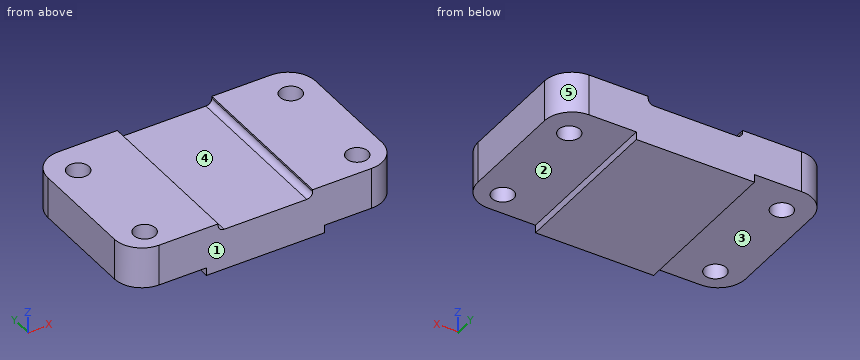
from build123d import *

# Parameters (mm, degrees)
F0_W     = 44
F0_H     = 82
F0_R     = 5.5
F0_W_2   = 48
F1_DEPTH = 12.5
F2_R     = 14
F3_W     = 48
F3_H     = 4
F4_DEPTH = 82.001
F5_R     = 3
F6_W     = 38
F6_H     = 4
F7_DEPTH = 82.001


with BuildPart() as f1:
    # F0 (on Top) → F1 (new body, symmetric)
    with BuildSketch(Plane.XY):
        with Locations((22, 41)):
            Rectangle(F0_W, F0_H)
        with Locations((14, 11.8173863739)):
            Circle(F0_R, mode=Mode.SUBTRACT)
        with Locations((14, 65.8173863739)):
            Circle(F0_R, mode=Mode.SUBTRACT)
        with Locations((68, 41)):
            Rectangle(F0_W_2, F0_H)
        with Locations((114, 41)):
            Rectangle(F0_W, F0_H)
        with Locations((122, 11.8173863739)):
            Circle(F0_R, mode=Mode.SUBTRACT)
        with Locations((122, 65.8173863739)):
            Circle(F0_R, mode=Mode.SUBTRACT)
    extrude(amount=F1_DEPTH, both=True)

    # F2
    f2_edges = [f1.edges().sort_by_distance(p)[0] for p in [
        (0, 82, 0),
        (136, 82, 0),
        (136, 0, 0),
        (0, 0, 0),
    ]]
    fillet(f2_edges, radius=F2_R)

    # F3 (on face) → F4 (cut, through all)
    with BuildSketch(Plane.XZ):
        with Locations((68, 10.5)):
            Rectangle(F3_W, F3_H)
    extrude(amount=-F4_DEPTH, mode=Mode.SUBTRACT)

    # F5
    f5_edges = [f1.edges().sort_by_distance(p)[0] for p in [
        (44, 41, 8.5),
        (92, 41, 8.5),
    ]]
    fillet(f5_edges, radius=F5_R)

    # F6 (on face) → F7 (cut, through all)
    with BuildSketch(Plane.XZ):
        with Locations((117, -10.5)):
            Rectangle(F6_W, F6_H)
        with Locations((19, -10.5)):
            Rectangle(F6_W, F6_H)
    extrude(amount=-F7_DEPTH, mode=Mode.SUBTRACT)


solid = f1.part
Geometry: final body of the model. Coordinates: model frame, mm. Face numbers are marked on the shaded views. A direction names the side the tool comes from. Coordinates: 2 decimals unless noted, no trailing zeros. Loops run counter-clockwise (first coordinate to the right, second up) from the corner with the lowest first, then second, coordinate; pieces in that order, holes last. Notation, with made-up numbers: M 24,46 L 38,46 A7 cw 38,59 Z; hole C -1.5,75 d11. An arc over 180 degrees is marked long. One line per item, written item: value. Start each with the question number.
1) Material intervals for L1, parallel to Y at x = 122, z = 2.75; L2, parallel to X at y = 64.5, z = -6.25; L3, parallel to Y at x = 126.5, z = 6.5, sorted ascending. Write a range as from..to.
2) Pin query (flat end, axial travel): P1, Ø14.5, axis at x = 122, y = 11.82, coming from the -Z side; P2, Ø1.2, axis at y = 24, z = -10.5, coming from the -X side; P3, Ø12, axis at x = 91.5, z = -1, coming from the -Y side; P4, Ø10, axis at x = 14, y = 65.82, coming from the +Z side. Return the tip coordinate at first contact, or that it passes through.
3) Cut plane A-A (y = 32). Return loops of the section in (x, z).
4) Reachability of the marked faces 1, 2, 3, 4 and 5 from +Z, -Z, +X, -X, +Y, -Y: full face, straight path, thin tool, end or side. Return the list, or none.
5) Cut plane B-B (z = 6.25). Return loops of the section in (x, y), then the cut area to 3 significant figures.
6) Cut plane D-D (x = 63.5). Return loops of the section in (y, z).
7) Cut plane C-C (z = -11). Return loops of the section in (x, y), then the cut area to 3 significant figures.
Evaluation:
1. L1: 0..6.32, 17.32..60.32, 71.32..82
1. L2: 0..8.66, 19.34..116.66, 127.34..136
1. L3: 0.74..8.66, 14.98..62.66, 68.98..81.26
2. P1: z = -8.5
2. P2: x = 38
2. P3: y = 0
2. P4: through
3. outline: M 0,-8.5 L 38,-8.5 L 38,-12.5 L 98,-12.5 L 98,-8.5 L 136,-8.5 L 136,12.5 L 92,12.5 L 92,11.5 A3 cw 89,8.5 L 47,8.5 A3 cw 44,11.5 L 44,12.5 L 0,12.5 Z
4. face 1: +Z, -Z, +X, -X, -Y
4. face 2: -Z, +X, +Y, -Y
4. face 3: -Z, -X, +Y, -Y
4. face 4: +Z, +Y, -Y
4. face 5: +Z, -Z, +X, +Y
5. outline: M 0,14 A14 ccw 14,0 L 122,0 A14 ccw 136,14 L 136,68 A14 ccw 122,82 L 14,82 A14 ccw 0,68 Z; hole C 14,11.82 d11; hole C 14,65.82 d11; hole C 122,11.82 d11; hole C 122,65.82 d11
5. area: 10,600 mm^2
6. outline: M 0,-12.5 L 82,-12.5 L 82,8.5 L 0,8.5 Z
7. outline: M 38,0 L 98,0 L 98,82 L 38,82 Z
7. area: 4,920 mm^2
